Read the model definition and answer for the solid it produces. Units are mm, in the model's axes. Face numbers are marked on the shaded views. A direction names the side the tool comes from. Give positions to 0.01 mm unless a question says otherwise; leave off trailing zeros. Order: outer loops, then holes, each group sorted by start corner. A loop starts at its lowest first (then second) coordinate and runs counter-clockwise, first axis right, second up. Notation, with made-up numbers: (0.5, 76.25) - (50.5, 76.25) arc R11 cw to (50.5, 93.25) - close; hole circle Ø3 at (88, -32). An arc over 180 degrees is marked (long way). Write item = value, one per line.
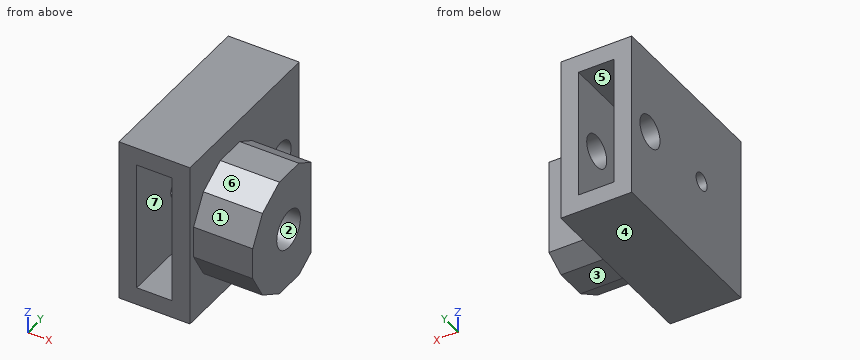
Autodesk Inventor part; units mm, degrees
ref_plane "YZ Plane" through (0, 0, 0) normal (1, 0, 0) x (0, 1, 0)
ref_plane "XZ Plane" through (0, 0, 0) normal (0, 1, 0) x (-1, 0, 0)
ref_plane "XY Plane" through (0, 0, 0) normal (0, 0, 1) x (1, 0, 0)
sketch "Sketch1" plane through (0, 0, 0) normal (0, 1, 0) x (-1, 0, 0)
  line L0 (0, 0) -> (6, 0)
  line L1 (6, 0) -> (6, -22)
  line L2 (6, -22) -> (0, -22)
  line L3 (0, -22) -> (0, 0)
  line L4 (9, 3) -> (-3, 3)
  line L5 (-3, 3) -> (-3, -25)
  line L6 (-3, -25) -> (9, -25)
  line L7 (9, -25) -> (9, 3)
  point P0 (3, 0)
  point P1 (3, -25)
  dimension "d0" = 22
  dimension "d1" = 6
  dimension "d2" = 3
  dimension "d3" = 3
  dimension "d4" = 3
  dimension "d5" = 3
extrude "Extrusion1" add sketch "Sketch1" along normal blind 30
sketch "Sketch2" plane through (3, 0, 3) normal (1, 0, 0) x (0, 0, -1)
  circle A0 centre (14, 25) radius 2.75
  line L0 (0, 30) -> (28, 30)
  point P0 (3, 0)
  dimension "d8" = 5.5
  dimension "d11" = 5
extrude "Extrusion2" cut sketch "Sketch2" against normal blind 30
sketch "Sketch3" plane through (3, 0, 3) normal (1, 0, 0) x (0, 0, -1)
  line L0 (6.6175, 3.6795) -> (3.938, 8.3205)
  line L1 (3.938, 8.3205) -> (3.938, 13.6795)
  line L2 (3.938, 13.6795) -> (6.6175, 18.3205)
  line L3 (6.6175, 18.3205) -> (11.2585, 21)
  line L4 (11.2585, 21) -> (16.6175, 21)
  line L5 (16.6175, 21) -> (21.2585, 18.3205)
  line L6 (21.2585, 18.3205) -> (23.938, 13.6795)
  line L7 (23.938, 13.6795) -> (23.938, 8.3205)
  line L8 (23.938, 8.3205) -> (21.2585, 3.6795)
  line L9 (21.2585, 3.6795) -> (16.6175, 1)
  line L10 (16.6175, 1) -> (11.2585, 1)
  line L11 (11.2585, 1) -> (6.6175, 3.6795)
  line L12 (0, 30) -> (28, 30)
  circle A0 centre (14, 10.8347) radius 3.253
  point P0 (3, 0)
  point P1 (13.938, 11)
  dimension "d12" = 10
  dimension "d13" = 19
extrude "Extrusion3" add sketch "Sketch3" along normal blind 10
sketch "Sketch5" plane through (3, 10.8347, -11) normal (1, 0, 0) x (0, 0, -1)
  circle A0 centre (0, 0) radius 1.5
  point P0 (-11, -10.8347)
  dimension "d18" = 3
extrude "Extrusion5" cut sketch "Sketch5" against normal blind 12
sketch "Sketch6" plane through (13, 0, 3) normal (1, 0, 0) x (0, 0, -1)
  line L0 (23, 22) -> (5, 22)
  line L1 (5, 22) -> (5, 17)
  line L2 (5, 17) -> (23, 17)
  line L3 (23, 17) -> (23, 22)
  line L4 (28, 0) -> (28, 30)
  line L5 (0, 0) -> (0, 30)
  line L6 (0, 30) -> (28, 30)
  point P0 (3, 0)
  dimension "d21" = 5
  dimension "d22" = 5
  dimension "d23" = 5
  dimension "d24" = 8
extrude "Extrusion6" cut sketch "Sketch6" against normal blind 10
equation "\"d22\" = d21"
properties part number "RollY" material "Thermoplastic Resin"
1. Flat-ended cylindrical pins translate along their axes: pin 1 (1.6 mm diameter, centred on x = 9.5, z = -10.5, fed in from -Y); pin 2 (6 mm diameter, centred on x = 8.5, y = 10, fed in from -Z); pin 3 (5 mm diameter, centred on y = 10.83, z = -11, fed in from +X). Find the tip coordinate at first contact, or state that the pin passes through.
Recorded:
pin_1 = 1
pin_2 = -20.94
pin_3 = 3
2. Section B-B (x = -2.75) is taken. Determine the outline of the cut face in (y, z).
Recorded:
outline = (0, -25) - (30, -25) - (30, -22) - (0, -22) - close; (0, 0) - (30, 0) - (30, 3) - (0, 3) - close
3. Section C-C (z = -11) is taken. Count the separate pieces of the cut face and the enclosed holes in it, and give its area (3 significant figures).
Recorded:
separate_pieces = 6
enclosed_holes = 0
area = 224 mm^2
4. Section D-D (y = 20.25) is taken. Determine the outline of the cut face in (x, z).
Recorded:
outline = (-9, -25) - (3, -25) - (3, 3) - (-9, 3) - close; hole (-6, -22) - (0, -22) - (0, 0) - (-6, 0) - close
5. Straight lines are drawn through the part: L1, parallel to Y at x = 1, z = -11; L2, parallel to Z at x = -2, y = 9; L3, parallel to X at y = 19.5, z = -19. For each, find the intervals that lie inside material, in ascending order. Write a range as [from, to].
Recorded:
L1 = [0, 9.33], [12.33, 22.25], [27.75, 30]
L2 = [-25, -22], [0, 3]
L3 = [-9, -6], [0, 3]
6. Determine the mould class of the marked faces 4, 5, 6 and 7 for opening direction Z: +Z half, -Z half, draft (parallel to the pull), parting line (faces both ways), or undercut.
Recorded:
face_4 = -Z half
face_5 = undercut
face_6 = +Z half
face_7 = undercut
7. Section A-A (y = 25) is taken. Determine the outline of the cut face in (x, z), and give its area (3 significant figures).
Recorded:
outline = (-9, -25) - (3, -25) - (3, -13.75) - (0, -13.75) - (0, -22) - (-6, -22) - (-6, -13.75) - (-9, -13.75) - close; (-9, -8.25) - (-6, -8.25) - (-6, 0) - (0, 0) - (0, -8.25) - (3, -8.25) - (3, 3) - (-9, 3) - close
area = 171 mm^2
8. For the marked faces 1, 2 and 3, determine the directions among +Z, -Z, +X, -X, +Y, -Y from which every point of the face is accessible in a straight line to the end or side of a thin tool.
Recorded:
face_1 = +Z, +X, -Y
face_2 = +X
face_3 = -Z, +X, +Y, -Y
